Input: part model. Units: mm. Frame: model coordinates. Coordinates: 2 decimals unless noted, no trailing zeros. Loops run counter-clockwise (first coordinate to the right, second up) from the corner with the lowest first, then second, coordinate; pieces in that order, holes last. Notation, with made-up numbers: (79.5, 12.5) -> (114.5, 12.5) arc R6 ccw to (114.5, 20.5) -> close; hole circle Ø7 at (39, -11). An arc over 180 degrees is marked (long way). Answer as a JSON object with one key per item and string values.
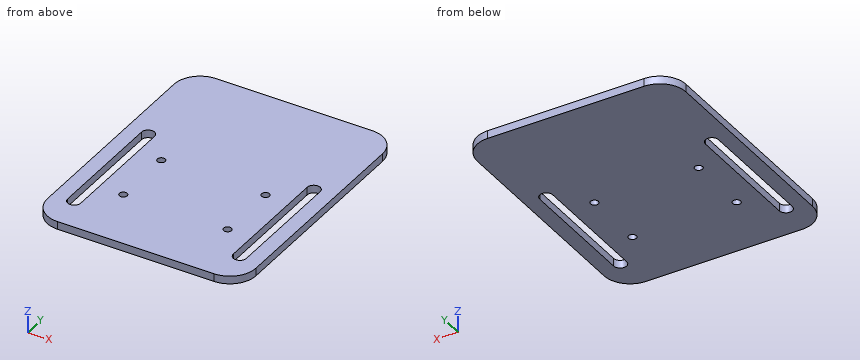
from build123d import *

# Parameters (mm, degrees)
F0_W     = 40
F0_H     = 100
F1_DEPTH = 3
F3_D     = 3
F5_DEPTH = 25
F6_R     = 10


with BuildPart() as f1:
    # F0 (on Top) → F1 (new body)
    with BuildSketch(Plane.XY):
        with Locations((20, 50)):
            Rectangle(F0_W, F0_H)
    extrude(amount=F1_DEPTH)

    # F3 (through all)
    with Locations(Plane(origin=(0, 0, 0), x_dir=(1, 0, 0), z_dir=(0, 0, -1))):
        with Locations((20, -49), (20, -25)):
            Hole(F3_D / 2)

    # F4 (on face) → F5 (cut)
    with BuildSketch(Plane.XY.offset(3)):
        with BuildLine():
            ThreePointArc((34.2711234093, 60.0486546755), (31.7711234093, 62.5486546755), (29.2711234093, 60.0486546755))
            Line((29.2711234093, 60.0486546755), (29.2711234093, 13.3645236492))
            ThreePointArc((29.2711234093, 13.3645236492), (31.7711234093, 10.8645236492), (34.2711234093, 13.3645236492))
            Line((34.2711234093, 13.3645236492), (34.2711234093, 60.0486546755))
        make_face()
    extrude(amount=-F5_DEPTH, mode=Mode.SUBTRACT)

    # F6
    f6_edges = [f1.edges().sort_by_distance(p)[0] for p in [
        (40, 100, 1.5),
        (40, 0, 1.5),
    ]]
    fillet(f6_edges, radius=F6_R)

    # F7: F1 across plane


with BuildPart() as f1_1:
    add(f1.part)
    add(f1.part.mirror(Plane.YZ))


solid = f1_1.part
1. Section query D-D (z = 0.6). Return loops of the section in (x, y).
Reply:
{"outline": "(-40, 10) arc R10 ccw to (-30, 0) -> (30, 0) arc R10 ccw to (40, 10) -> (40, 90) arc R10 ccw to (30, 100) -> (-30, 100) arc R10 ccw to (-40, 90) -> close; hole (-34.27, 13.36) arc R2.5 ccw to (-29.27, 13.36) -> (-29.27, 60.05) arc R2.5 ccw to (-34.27, 60.05) -> close; hole circle Ø3 at (-20, 25); hole circle Ø3 at (-20, 49); hole circle Ø3 at (20, 25); hole circle Ø3 at (20, 49); hole (29.27, 13.36) arc R2.5 ccw to (34.27, 13.36) -> (34.27, 60.05) arc R2.5 ccw to (29.27, 60.05) -> close"}
2. Pin query (flat end, axial travel): P1, Ø3.5, axis at x = 20, y = 49, coming from the +Z side; P2, Ø1.8, axis at x = -20, y = 25, coming from the -Z side. Return the tip coordinate at first contact, or that it passes through.
Reply:
{"P1": "stops at z = 3", "P2": "passes through"}
3. Line query: line 1 along Y through (x, z) = (-20, 2); line 2 along X through (y, z) = (25, 1.8); line 3 along X through (y, z) = (23, 2.5). Output: solid intervals per line, ascending.
Reply:
{"line 1": "y = 0 to 23.5, 26.5 to 47.5, 50.5 to 100", "line 2": "x = -40 to -34.27, -29.27 to -21.5, -18.5 to 18.5, 21.5 to 29.27, 34.27 to 40", "line 3": "x = -40 to -34.27, -29.27 to 29.27, 34.27 to 40"}
4. Section query B-B (x = -20). Return loops of the section in (y, z).
Reply:
{"outline": "(0, 0) -> (23.5, 0) -> (23.5, 3) -> (0, 3) -> close; (26.5, 0) -> (47.5, 0) -> (47.5, 3) -> (26.5, 3) -> close; (50.5, 0) -> (100, 0) -> (100, 3) -> (50.5, 3) -> close"}
5. Section query A-A (y = 49). Return loops of the section in (x, z).
Reply:
{"outline": "(-40, 0) -> (-34.27, 0) -> (-34.27, 3) -> (-40, 3) -> close; (-29.27, 0) -> (-21.5, 0) -> (-21.5, 3) -> (-29.27, 3) -> close; (-18.5, 0) -> (18.5, 0) -> (18.5, 3) -> (-18.5, 3) -> close; (21.5, 0) -> (29.27, 0) -> (29.27, 3) -> (21.5, 3) -> close; (34.27, 0) -> (40, 0) -> (40, 3) -> (34.27, 3) -> close"}
6. Section query C-C (y = 29.5). Return loops of the section in (x, z).
Reply:
{"outline": "(-40, 0) -> (-34.27, 0) -> (-34.27, 3) -> (-40, 3) -> close; (-29.27, 0) -> (29.27, 0) -> (29.27, 3) -> (-29.27, 3) -> close; (34.27, 0) -> (40, 0) -> (40, 3) -> (34.27, 3) -> close"}
